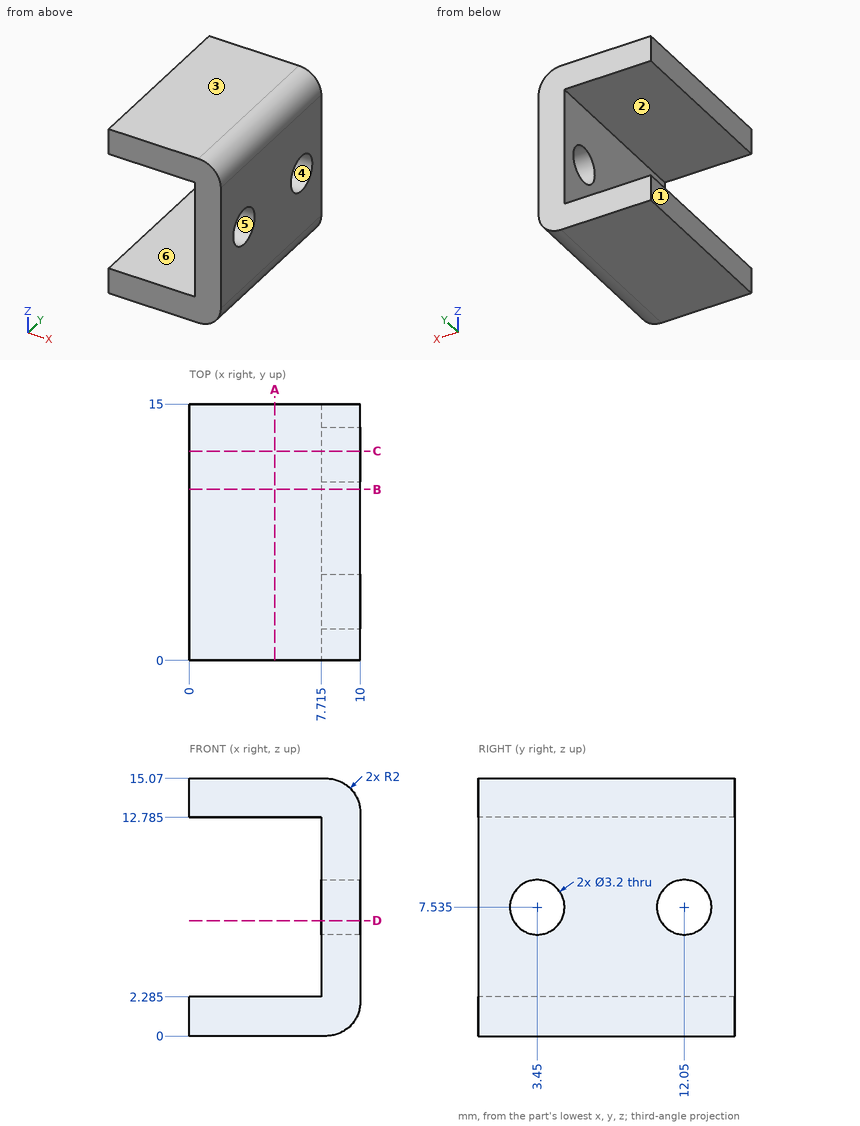
Answer from the drawing. Dimensions are ordinates in mm from the lowest x, y and z of the part. A direction names the side the tool comes from. Give positions to 0.01 mm unless a question says otherwise; leave off trailing zeros. Write each loop counter-clockwise with the first axis right and the second up, starting at its lowest first coordinate (ties: lowest second). Pieces come first, ordered by that corner, then holes.
1) For a pull along Z with two mould halves and no side action, classify the marked faces 1, 2, 3 and 4 as pulls with the +Z half, pulls with the -Z half, needs draft (parallel to the pull), parting line crosses it, or undercut.
2) Section C-C (y = 12.25) is taken. Write down the section's boundary in (x, z) (1 decimal).
3) Find the intervals of material crossed by L1, parallel to Z at x = 3.5, y = 2.5 (3 decimals); L2, parallel to X at y = 5, z = 12.5 (3 decimals); L3, parallel to Z at x = 8.75, y = 4.5, in increasing order.
4) Given P1, Ø5.5, axis at y = 10, z = 9, coming from the -X side (3 decimals), flat-ended and moving along its own axis, determine where the tip first touches the part or whether it passes through.
5) Section A-A (x = 5) is taken. Write down the section's boundary in (y, z) (3 decimals).
6) Section B-B (y = 10) is taken. Write down the section's boundary in (x, z) (3 decimals), and give its area (3 significant figures).
7) Section D-D (z = 6.75) is taken. Write down the section's boundary in (x, y) (1 decimal), and give its area (3 significant figures).
8) A tool of negligible diameter and unlimited length cuts with its end or side. For the marked faces 5 and 6, from which of +Z, -Z, +X, -X, +Y, -Y can it reach the whole face along a straight path? Write none if from no direction.
Response:
1. face 1: needs draft
1. face 2: undercut
1. face 3: pulls with the +Z half
1. face 4: undercut
2. outline: (0, 0) - (8, 0) arc R2 ccw to (10, 2) - (10, 5.9) - (7.7, 5.9) - (7.7, 2.3) - (0, 2.3) - close; (0, 12.8) - (7.7, 12.8) - (7.7, 9.1) - (10, 9.1) - (10, 13.1) arc R2 ccw to (8, 15.1) - (0, 15.1) - close
3. L1: z = 0 to 2.285, 12.785 to 15.07
3. L2: x = 7.715 to 10
3. L3: z = 0.15 to 6.33, 8.74 to 14.92
4. P1: stops at x = 7.715
5. outline: (0, 0) - (15, 0) - (15, 2.285) - (0, 2.285) - close; (0, 12.785) - (15, 12.785) - (15, 15.07) - (0, 15.07) - close
6. outline: (0, 0) - (8, 0) arc R2 ccw to (10, 2) - (10, 13.07) arc R2 ccw to (8, 15.07) - (0, 15.07) - (0, 12.785) - (7.715, 12.785) - (7.715, 2.285) - (0, 2.285) - close
6. area: 68.0 mm2
7. outline: (7.7, 0) - (10, 0) - (10, 2.1) - (7.7, 2.1) - close; (7.7, 4.8) - (10, 4.8) - (10, 10.7) - (7.7, 10.7) - close; (7.7, 13.4) - (10, 13.4) - (10, 15) - (7.7, 15) - close
7. area: 21.5 mm2
8. face 5: +X, -X
8. face 6: -X, +Y, -Y
